Geometry check sheet. Reference: the model listing, model coordinates, mm. A direction names the side the tool comes from. Give positions to 0.01 mm unless a question says otherwise; leave off trailing zeros. Write each loop counter-clockwise with the first axis right and the second up, starting at its lowest first coordinate (ties: lowest second). Pieces come first, ordered by that corner, then holes. Notation, with made-up numbers: (39.5, -28.5) - (62.5, -28.5) arc R12 cw to (62.5, -11.5) - close; hole circle Ø2 at (66.5, 71.5). An arc over 180 degrees is marked (long way). Use a Markdown table: item, result.
Autodesk Inventor part; units mm, degrees
ref_plane "YZ Plane" through (0, 0, 0) normal (1, 0, 0) x (0, 1, 0)
ref_plane "XZ Plane" through (0, 0, 0) normal (0, 1, 0) x (-1, 0, 0)
ref_plane "XY Plane" through (0, 0, 0) normal (0, 0, 1) x (1, 0, 0)
sketch "Sketch1" plane through (0, 0, 0) normal (0, 1, 0) x (-1, 0, 0)
  line L0 (0, 0) -> (0, -34)
  line L1 (0, -34) -> (8, -34)
  line L2 (8, -34) -> (8, 0)
  line L3 (8, 0) -> (0, 0)
  line L4 (23, -34) -> (23, -27)
  line L5 (23, -27) -> (8, -27)
  line L6 (23, 0) -> (23, -7)
  line L7 (23, -7) -> (8, -7)
  line L8 (8, -7) -> (8, -27)
  line L9 (8, -17) -> (4, -17)
  line L10 (4, -17) -> (4, -22)
  line L11 (4, -17) -> (4, -12)
  circle A0 centre (4, -12) radius 1.6
  circle A1 centre (4, -22) radius 1.6
  line L12 (8, -7) -> (0, -7)
  line L13 (8, -27) -> (0, -27)
  line L14 (23, -7) -> (23, -2)
  circle A2 centre (15.5, -2) radius 2.6
  arc A3 (18.9641, 0) -> (12.0359, 0) centre (15.5, -2) ccw
  line L15 (8, 0) -> (12.0359, 0)
  line L16 (18.9641, 0) -> (23, 0)
  line L17 (23, -27) -> (23, -32)
  circle A4 centre (15.5, -32) radius 2.6
  arc A5 (12.0359, -34) -> (18.9641, -34) centre (15.5, -32) ccw
  line L18 (8, -34) -> (12.0359, -34)
  line L19 (18.9641, -34) -> (23, -34)
  circle A6 centre (4, -12) radius 3
  circle A7 centre (4, -22) radius 3
  dimension "d0" = 34
  dimension "d1" = 8
  dimension "d2" = 15
  dimension "d3" = 7
  dimension "d4" = 15
  dimension "d5" = 7
  dimension "d6" = 4
  dimension "d7" = 5
  dimension "d8" = 5
  dimension "d9" = 3.2
  dimension "d10" = 3.2
  dimension "d11" = 5
  dimension "d12" = 5.2
  dimension "d13" = 8
  dimension "d14" = 5
  dimension "d15" = 5.2
  dimension "d16" = 8
  dimension "d21" = 6
  dimension "d22" = 6
extrude "Extrusion1" add sketch "Sketch1" along normal blind 9 contours L3 L2 L12 L0 | L12 L2 L13 L0 | L13 L2 L1 L0 | A6 | A7
extrude "Extrusion2" add sketch "Sketch1" along normal blind 15 contours L15 A3 L16 L6 L7 L2 | L5 L4 L19 A5 L18 L2
extrude "Extrusion3" cut sketch "Sketch1" along normal blind 4 contours A6 | A7
fillet "Fillet1" radius 2 2 edges at (-1, 4, -22) (-1, 4, -12)
properties part number "servo_holder"
1) Section check B-B on z = -32. Record the boundary of the cut face in (x, y), then the cut area to 3 significant figures.
Working result:
| item | result |
|---|---|
| outline | (-23, 0) - (-18.1, 0) - (-18.1, 15) - (-23, 15) - close; (-12.9, 0) - (0, 0) - (0, 9) - (-8, 9) - (-8, 15) - (-12.9, 15) - close |
| area | 219 mm² |
2) Section check C-C on x = -9.5. Record the boundary of the cut face in (y, z), then the cut area to 3 significant figures.
Working result:
| item | result |
|---|---|
| outline | (0, -34) - (15, -34) - (15, -27) - (0, -27) - close; (0, -7) - (15, -7) - (15, 0) - (0, 0) - close |
| area | 210 mm² |
3) Material ranges on L1, parallel to Z at x = -4, y = 0.65; L2, parallel to X at y = 1.35, z = -22; L3, parallel to Z at x = -14, y = 9.75, recorded low to high. Write a range as from..to.
Working result:
| item | result |
|---|---|
| L1 | z = -34..-25, -19..-15, -9..0 |
| L2 | x = -8..-7, -1..0 |
| L3 | z = -35.71..-34.12, -29.88..-27, -7..-4.12, 0.12..1.71 |
4) Set-up check for faces 1 (the flat face through (-8, 4, -17)), 2 (the cylindrical face through (-1, 1, -22)), 3 (the flat face through (-4, 9, -17)): record each of +Z, -Z, +X, -X, +Y, -Y from which the full face is reachable in a straight line by a thin tool's end or side.
Working result:
| item | result |
|---|---|
| face 1 | -X, +Y, -Y |
| face 2 | -Y |
| face 3 | +Z, -Z, +X, +Y |
5) Depth check by flat-ended pin: P1, Ø8.5, axis at x = -15.5, z = -2, coming from the -Y side; P2, Ø4, axis at x = -20.5, y = 13, coming from the +Z side; P3, Ø1.2, axis at x = -21, y = 5, coming from the +Z side; P4, Ø3, axis at y = 7, z = -24, coming from the -X side. Enter the tip coordinate at first touch or a pass-through.
Working result:
| item | result |
|---|---|
| P1 | stops at y = 0 |
| P2 | stops at z = 0.65 |
| P3 | stops at z = 0 |
| P4 | stops at x = -8 |
6) Mould release check, pull along X, two halves, no side actions. Record for faces 4 (the flat face through (-23, 7, -3)), 5 (the flat face through (-17.1, 15, -4.4)), 6 (the cylindrical face through (-15.4, 7.4, 2)), 7 (the cylindrical face through (-3.792, 6.465, -13.586)): pulls with the +X half, pulls with the -X half, needs draft (parallel to the pull), parting line crosses it, or undercut.
Working result:
| item | result |
|---|---|
| face 4 | pulls with the -X half |
| face 5 | needs draft |
| face 6 | parting line crosses it |
| face 7 | undercut |
7) Section check A-A on y = 11.5. Record the boundary of the cut face in (x, z), then the cut area to 3 significant figures.
Working result:
| item | result |
|---|---|
| outline | (-23, -34) - (-18.96, -34) arc R4 ccw to (-12.04, -34) - (-8, -34) - (-8, -27) - (-23, -27) - close; (-23, -7) - (-8, -7) - (-8, 0) - (-12.04, 0) arc R4 ccw to (-18.96, 0) - (-23, 0) - close; hole circle Ø5.2 at (-15.5, -32); hole circle Ø5.2 at (-15.5, -2) |
| area | 187 mm² |
8) Section check D-D on y = 1.5. Record the boundary of the cut face in (x, z), then the cut area to 3 significant figures.
Working result:
| item | result |
|---|---|
| outline | (-23, -34) - (-18.96, -34) arc R4 ccw to (-12.04, -34) - (0, -34) - (0, 0) - (-12.04, 0) arc R4 ccw to (-18.96, 0) - (-23, 0) - (-23, -7) - (-8, -7) - (-8, -27) - (-23, -27) - close; hole circle Ø5.2 at (-15.5, -32); hole circle Ø5.2 at (-15.5, -2); hole circle Ø6 at (-4, -22); hole circle Ø6 at (-4, -12) |
| area | 403 mm² |
